Design review of the part built by this model. Coordinates are the model's own, in mm. A direction names the side the tool comes from. Coordinates: 2 decimals unless noted, no trailing zeros. Loops run counter-clockwise (first coordinate to the right, second up) from the corner with the lowest first, then second, coordinate; pieces in that order, holes last. Notation, with made-up numbers: M -16,86 L 32,86 A34 ccw 32,119 Z; hole C 72,10.25 d10. An arc over 180 degrees is marked long. One line per item, written item: value.
```python
from build123d import *

# Parameters (mm, degrees)
EXTRUDE_1_DEPTH     = 50
CUT_EXTRUDE_START   = -50
SKETCH_2_W          = 99.785929991
SKETCH_2_H          = 100
CUT_EXTRUDE_1_DEPTH = 50
SKETCH_7_W          = 19.044434788
SKETCH_7_H          = 15
CUT_EXTRUDE_5_DEPTH = 15
SKETCH_9_R          = 5
CUT_EXTRUDE_6_DEPTH = 10


with BuildPart() as part:
    # 草图1 → 凸台-拉伸1 (new, symmetric)
    with BuildSketch(Plane(origin=(0, 0, 0), x_dir=(1, 0, 0), z_dir=(0, 1, 0))):
        with BuildLine():
            Line((0, 7.5), (75, 7.5))
            ThreePointArc((75, 7.5), (85.606601718, 11.893398282), (90, 22.5))
            Line((90, 22.5), (90, 82.5))
            Line((90, 82.5), (105, 82.5))
            Line((105, 82.5), (105, 22.5))
            ThreePointArc((105, 22.5), (96.213203436, 1.286796564), (75, -7.5))
            Line((75, -7.5), (0, -7.5))
            ThreePointArc((0, -7.5), (-7.5, 0), (0, 7.5))
        make_face()
    extrude(amount=EXTRUDE_1_DEPTH, both=True)

    # 草图2 → 切除-拉伸1 (cut)
    with BuildSketch(Plane(origin=(0, 25, 0), x_dir=(1, 0, 0), z_dir=(0, 1, 0)).offset(CUT_EXTRUDE_START)):
        with Locations((64.892964996, 39.075948396)):
            Rectangle(SKETCH_2_W, SKETCH_2_H)
    extrude(amount=CUT_EXTRUDE_1_DEPTH, mode=Mode.SUBTRACT)

    # 草图7 → 切除-拉伸5 (cut)
    with BuildSketch(Plane(origin=(0, 50, 0), x_dir=(1, 0, 0), z_dir=(0, 1, 0))):
        with Locations((-2.022217394, 0)):
            Rectangle(SKETCH_7_W, SKETCH_7_H)
    cut_extrude_5 = extrude(amount=-CUT_EXTRUDE_5_DEPTH, mode=Mode.SUBTRACT)

    # 镜向1: 切除-拉伸5 across plane
    add(cut_extrude_5.mirror(Plane.ZX), mode=Mode.SUBTRACT)

    # 草图9 → 切除-拉伸6 (cut)
    with BuildSketch(Plane(origin=(0, 35, 0), x_dir=(1, 0, 0), z_dir=(0, 1, 0))):
        with BuildLine():
            Line((0, 7.5), (7.5, 7.5))
            Line((7.5, 7.5), (7.5, -7.5))
            Line((7.5, -7.5), (0, -7.5))
            ThreePointArc((0, -7.5), (-7.5, 0), (0, 7.5))
        make_face()
        with Locations(Location((0, 0, 0), (0, 0, 270))):
            Circle(SKETCH_9_R, mode=Mode.SUBTRACT)
    cut_extrude_6 = extrude(amount=-CUT_EXTRUDE_6_DEPTH, mode=Mode.SUBTRACT)

    # 镜向2: 切除-拉伸6 across plane
    add(cut_extrude_6.mirror(Plane.ZX), mode=Mode.SUBTRACT)


solid = part.part
```
(1) Tool access review of faces 5 (the flat face through (90, 38, -52)), 6 (the flat face through (83, 25, -8)), 7 (the flat face through (7.5, 38, 0)), 8 (the flat face through (85, -50, -11)), 9 (the cylindrical face through (-4.88, 30.07, -1.08)): name each direction out of +Z, -Z, +X, -X, +Y, -Y from which nothing blocks a thin tool from reaching the whole face with its end or side.
Reply:
face 5: -Z, -X, +Y, -Y
face 6: +Z, -Z, +X
face 7: +Z, -Z, +Y
face 8: +Z, -Z, +X, -X, -Y
face 9: +Y
(2) We need section A-A on y = 28. State the section outline as (x, z) points.
Reply:
outline: C 0,0 d10; M 7.5,-7.5 L 75,-7.5 A15 cw 90,-22.5 L 90,-82.5 L 105,-82.5 L 105,-22.5 A30 ccw 75,7.5 L 7.5,7.5 Z
(3) We need section C-C on z = -17. State the section outline as (x, y) points, then the cut area to 3 significant figures.
Reply:
outline: M 88.96,-50 L 104.49,-50 L 104.49,-25 L 88.96,-25 Z; M 88.96,25 L 104.49,25 L 104.49,50 L 88.96,50 Z
area: 777 mm2
(4) Mouldability with a two-part tool opening along Y and no side actions: class faces 1 (the flat face through (15, 0, 0)), 2 (the flat face through (83, -25, -8)), 3 (the flat face through (7.5, -38, 0)), 4 (the flat face through (5, 25, 2)) as released by +Y, released by -Y, zero draft, split by the parting line, or undercut.
Reply:
face 1: undercut
face 2: undercut
face 3: zero draft
face 4: released by +Y
(5) We need section D-D on y = -40.5. State the section outline as (x, z) points, then the cut area to 3 significant figures.
Reply:
outline: M 7.5,-7.5 L 75,-7.5 A15 cw 90,-22.5 L 90,-82.5 L 105,-82.5 L 105,-22.5 A30 ccw 75,7.5 L 7.5,7.5 Z
area: 2,440 mm2
(6) To check wall thickness, follow line 1 along Z through (x, y) = (0.5, -6.5); line 2 along X through (y, z) = (-30, -1); line 3 along X through (y, z) = (-39, -72.5). State the ranges of each line that lie inside material, in increasing order. Write a range as [from, to].
Reply:
line 1: z = [-7.5, 7.5]
line 2: x = [-4.9, 4.9], [7.5, 95.92]
line 3: x = [90, 105]
(7) Insertion check: pin 1 (5 mm diameter, centred on x = 56, y = 26, fed in from -Z); pin 2 (4.5 mm diameter, centred on x = -2.5, z = 3, fed in from +Y); pin 3 (4.5 mm diameter, centred on x = -1.5, z = -2, fed in from -Y). Each pin has a flat end and moves straight along its axis. Give the tip position at first contact, or say it passes through.
Reply:
pin 1: stops at z = -7.5
pin 2: stops at y = 35
pin 3: stops at y = -35
(8) We need section B-B on x = 45.5. State the section outline as (y, z) points, then the cut area to 3 significant figures.
Reply:
outline: M -50,-7.5 L -25,-7.5 L -25,7.5 L -50,7.5 Z; M 25,-7.5 L 50,-7.5 L 50,7.5 L 25,7.5 Z
area: 750 mm2
